from build123d import *

# Parameters (mm, degrees)
ESQUISSE1_W             = 233
ESQUISSE1_H             = 300
BOSS_EXTRU_1_DEPTH      = 4.2
ESQUISSE2_R             = 2.55
ENL_V_MAT_EXTRU_1_DEPTH = 5.2


with BuildPart() as part:
    # Esquisse1 → Boss.-Extru.1 (new body)
    with BuildSketch(Plane.XY):
        with Locations((-3.063037439, -81.267653759)):
            Rectangle(ESQUISSE1_W, ESQUISSE1_H)
    extrude(amount=BOSS_EXTRU_1_DEPTH)

    # Esquisse2 → Enlèv. mat.-Extru.1 (cut, through all)
    with BuildSketch(Plane.XY.offset(4.2)):
        with Locations((-78.063037439, -197.267653759)):
            Circle(ESQUISSE2_R)
        with Locations((-1.063037439, -197.267653759)):
            Circle(ESQUISSE2_R)
        with BuildLine():
            Line((-69.563037439, -231.267653759), (-9.563037439, -231.267653759))
            ThreePointArc((-9.563037439, -231.267653759), (-39.563037439, -201.267653759), (-69.563037439, -231.267653759))
        make_face()
    extrude(amount=-ENL_V_MAT_EXTRU_1_DEPTH, mode=Mode.SUBTRACT)


solid = part.part
Work out the finished part from the listing and answer in its coordinate system (mm). Round coordinates to 2 decimals unless told otherwise and drop trailing zeros. Write each loop counter-clockwise with the first axis right and the second up, starting at its lowest first coordinate (ties: lowest second). Pieces come first, ordered by that corner, then holes. Notation, with made-up numbers: (8.25, 51) - (21.25, 51) arc R19 cw to (21.25, 82) - close; hole circle Ø4 at (61, 59). An arc over 180 degrees is marked (long way). Answer in a Markdown table with one row per item. Add a question column.
1. A cutting plane is placed at B-B, the plane x = -37. Determine the outline of the cut face in (y, z).
2. Given pin 1 (3 mm diameter, centred on x = -78.06, y = -197.27, fed in from -Z), flat-ended and moving along its own axis, determine where the tip first touches the part or whether it passes through.
3. Find the intervals of material crossed by line 1 along Y through (x, z) = (-0.5, 3); line 2 along X through (y, z) = (-210, 2); line 3 along Y through (x, z) = (-22, 1.65), in increasing order. Write a range as from..to.
4. A cutting plane is placed at A-A, the plane z = 2.65. Determine the outline of the cut face in (x, y).
5. The mould has two halves that part along X. Classify faces 1 (the cylindrical face through (-38.903, -201.275, 2.129)), 2 (the flat face through (-5, -79, 4.2)): +X half, -X half, draft (parallel to the pull), parting line (faces both ways), or undercut.
Worked out:
| question | item | result |
|---|---|---|
| 1 | outline | (-201.38, 0) - (68.73, 0) - (68.73, 4.2) - (-201.38, 4.2) - close |
| 2 | pin 1 | through |
| 3 | line 1 | -231.27..-199.75, -194.78..68.73 |
| 3 | line 2 | -119.56..-60.72, -18.4..113.44 |
| 3 | line 3 | -206.95..68.73 |
| 4 | outline | (-119.56, -231.27) - (-69.56, -231.27) arc R30 cw to (-9.56, -231.27) - (113.44, -231.27) - (113.44, 68.73) - (-119.56, 68.73) - close; hole circle Ø5.1 at (-78.06, -197.27); hole circle Ø5.1 at (-1.06, -197.27) |
| 5 | face 1 | undercut |
| 5 | face 2 | draft |
